The model under review builds one solid part; all positions refer to its coordinate system, in mm. Face numbers are marked on the shaded views. A direction names the side the tool comes from. Coordinates: 2 decimals unless noted, no trailing zeros. Loops run counter-clockwise (first coordinate to the right, second up) from the corner with the lowest first, then second, coordinate; pieces in that order, holes last. Notation, with made-up numbers: (25.25, 19.5) - (30.25, 19.5) arc R26 cw to (30.25, 35.5) - close; hole circle Ø3 at (82.25, -28). An arc over 180 degrees is marked (long way). Answer in a Markdown table with one row per item. Add a question column.
(1) For line 1 along X through (y, z) = (10.25, 0); line 2 along Z through (x, y) = (0, 0.5); line 3 along Z through (x, y) = (-2, 1.25), list the stretches that pass through material, from the lowest coordinate up.
(2) We need section C-C on y = 1.5. Write out the cut boundary in (x, z), plus the area to 3 significant figures.
(3) For P1, Ø10, axis at y = 5.5, z = 0.5, coming from the +X side; P2, Ø2, axis at x = 0.5, y = 3, coming from the -Z side; P3, Ø3.5, axis at y = 9.5, z = 1, coming from the -X side, all flat-tipped, find the tip position at first contact; note any pin that passes through.
(4) We need section B-B on x = 0. Write out the cut boundary in (y, z).
(5) We need section A-A on z = 0. Write out the cut boundary in (x, y).
(6) Mouldability with a two-part tool opening along Z and no side actions: class the marked faces 1, 2 and 3 as +Z half, -Z half, draft (parallel to the pull), parting line (faces both ways), or undercut.
(7) Machinability: for the marked faces 4, 5, 6, 7 and 8, which of the approach directions +Z, -Z, +X, -X, +Y, -Y give a long, thin tool a straight path to every point of the face, cutting with its end or side? Answer none if there is none.
(8) We need section D-D on x = -6. Write out the cut boundary in (y, z).
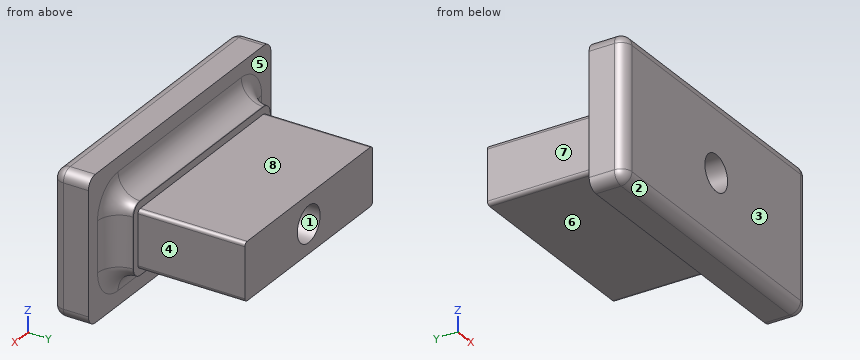
from build123d import *

# Parameters (mm, degrees)
SKETCH_W     = 30
SKETCH_H     = 10
PAD_DEPTH    = 3.1
SKETCH001_W  = 40
SKETCH001_H  = 20
PAD001_DEPTH = 5
FILLET_R     = 1.5
FILLET001_R  = 3
FILLET002_R  = 1.5
SKETCH002_W  = 28
SKETCH002_H  = 8
PAD002_DEPTH = 14.9
FILLET003_R  = 0.5
SKETCH003_R  = 2.5
POCKET_DEPTH = 25


with BuildPart() as part:
    # Sketch → Pad (new body)
    with BuildSketch(Plane.XZ):
        Rectangle(SKETCH_W, SKETCH_H)
    extrude(amount=PAD_DEPTH)

    # Sketch001 (on Face6 of Pad) → Pad001 (join)
    with BuildSketch(Plane.XZ.offset(3.1)):
        Rectangle(SKETCH001_W, SKETCH001_H)
    extrude(amount=PAD001_DEPTH)

    # Fillet
    fillet_edges = [part.edges().sort_by_distance(p)[0] for p in [
        (15, -1.55, 5),
        (15, -1.55, -5),
        (-15, -1.55, 5),
        (-15, -1.55, -5),
    ]]
    fillet(fillet_edges, radius=FILLET_R)

    # Fillet001
    fillet001_edges = [part.edges().sort_by_distance(p)[0] for p in [
        (0, -3.1, 5),
    ]]
    fillet(fillet001_edges, radius=FILLET001_R)

    # Fillet002
    fillet002_edges = [part.edges().sort_by_distance(p)[0] for p in [
        (0, -8.1, 10),
        (-20, -8.1, 0),
        (20, -8.1, 0),
        (0, -8.1, -10),
        (20, -5.6, 10),
        (-20, -5.6, 10),
        (20, -5.6, -10),
        (-20, -5.6, -10),
    ]]
    fillet(fillet002_edges, radius=FILLET002_R)

    # Sketch002 (on Face4 of Fillet001) → Pad002 (join)
    with BuildSketch(Plane(origin=(0, 0, 0), x_dir=(1, 0, 0), z_dir=(0, 1, 0))):
        Rectangle(SKETCH002_W, SKETCH002_H)
    extrude(amount=PAD002_DEPTH)

    # Fillet003
    fillet003_edges = [part.edges().sort_by_distance(p)[0] for p in [
        (14, 7.45, 4),
        (-14, 7.45, 4),
        (-14, 7.45, -4),
        (14, 7.45, -4),
    ]]
    fillet(fillet003_edges, radius=FILLET003_R)

    # Sketch003 (on Face18 of Fillet003) → Pocket (cut)
    with BuildSketch(Plane(origin=(0, 14.9, 0), x_dir=(1, 0, 0), z_dir=(0, 1, 0))):
        Circle(SKETCH003_R)
    extrude(amount=-POCKET_DEPTH, mode=Mode.SUBTRACT)


solid = part.part
Outcome:
| question | item | result |
|---|---|---|
| 1 | line 1 | -14 to -2.5, 2.5 to 14 |
| 1 | line 2 | -4 to -2.5, 2.5 to 4 |
| 1 | line 3 | -4 to -1.5, 1.5 to 4 |
| 2 | outline | (-14, -3.5) arc R0.5 ccw to (-13.5, -4) - (13.5, -4) arc R0.5 ccw to (14, -3.5) - (14, 3.5) arc R0.5 ccw to (13.5, 4) - (-13.5, 4) arc R0.5 ccw to (-14, 3.5) - close; hole circle Ø5 at (0, 0) |
| 2 | area | 204 mm² |
| 3 | P1 | x = 14 |
| 3 | P2 | z = -4 |
| 3 | P3 | x = -14 |
| 4 | outline | (-8.1, -8.5) arc R1.5 ccw to (-6.6, -10) - (-3.1, -10) - (-3.1, -8) arc R3 cw to (-0.1, -5) - (0, -5) - (0, -4) - (14.9, -4) - (14.9, -2.5) - (-8.1, -2.5) - close; (-8.1, 2.5) - (14.9, 2.5) - (14.9, 4) - (0, 4) - (0, 5) - (-0.1, 5) arc R3 cw to (-3.1, 8) - (-3.1, 10) - (-6.6, 10) arc R1.5 ccw to (-8.1, 8.5) - close |
| 5 | outline | (-20, -6.6) arc R1.5 ccw to (-18.5, -8.1) - (-2.5, -8.1) - (-2.5, 14.9) - (-14, 14.9) - (-14, 0) - (-15, 0) - (-15, -0.1) arc R3 cw to (-18, -3.1) - (-20, -3.1) - close; (2.5, -8.1) - (18.5, -8.1) arc R1.5 ccw to (20, -6.6) - (20, -3.1) - (18, -3.1) arc R3 cw to (15, -0.1) - (15, 0) - (14, 0) - (14, 14.9) - (2.5, 14.9) - close |
| 6 | face 1 | undercut |
| 6 | face 2 | -Z half |
| 6 | face 3 | draft |
| 7 | face 4 | +Z, -Z, +X, +Y |
| 7 | face 5 | +Y |
| 7 | face 6 | -Z, +X, -X, +Y |
| 7 | face 7 | +Z, -Z, -X, +Y |
| 7 | face 8 | +Z, +X, -X, +Y |
| 8 | outline | (-8.1, -8.5) arc R1.5 ccw to (-6.6, -10) - (-3.1, -10) - (-3.1, -8) arc R3 cw to (-0.1, -5) - (0, -5) - (0, -4) - (14.9, -4) - (14.9, 4) - (0, 4) - (0, 5) - (-0.1, 5) arc R3 cw to (-3.1, 8) - (-3.1, 10) - (-6.6, 10) arc R1.5 ccw to (-8.1, 8.5) - close |
